Model file for the job. Use its own axes, mm. Coordinates: 2 decimals unless noted, no trailing zeros. Write each loop counter-clockwise with the first axis right and the second up, starting at its lowest first coordinate (ties: lowest second). Pieces come first, ordered by that corner, then holes.
Q1. Drill centre lines: probe 1 along Y at (x, z) = (4, -2.5); probe 2 along Z at (x, y) = (1.1, 160); probe 3 along Z at (x, y) = (3.9, 202.5). Where is each one in solid material? Low to high.
Q2. Pull direction Z, two halves, no side cores. Call faces 1 (the flat face through (2.5, 101, -75)), 2 (the flat face through (3, 104, -80)), 3 (the flat face through (0, 104, -39)): released by +Z, released by -Z, zero draft, split by the parting line, or undercut.
Q3. Band-saw the part on A-A, the plane y = 84. Write the cut outline in (x, z).
Autodesk Inventor part; units mm, degrees
ref_plane "YZ Plane" through (0, 0, 0) normal (1, 0, 0) x (0, 1, 0)
ref_plane "XZ Plane" through (0, 0, 0) normal (0, 1, 0) x (-1, 0, 0)
ref_plane "XY Plane" through (0, 0, 0) normal (0, 0, 1) x (1, 0, 0)
sketch "Sketch1" plane through (0, 0, 0) normal (1, 0, 0) x (0, 1, 0)
  line L0 (0, 0) -> (205, 0)
  line L1 (205, 0) -> (205, -70)
  line L2 (205, -70) -> (0, -70)
  line L3 (0, -70) -> (0, 0)
  circle A0 centre (40, -2.5) radius 1
  circle A1 centre (80, -2.5) radius 1
  circle A2 centre (120, -2.5) radius 1
  circle A3 centre (160, -2.5) radius 1
  line L4 (0, 0) -> (0, 5)
  circle A4 centre (202.5, -2.5) radius 1.1944
  line L5 (0, -35) -> (205, -35) construction
  point P0 (40, -67.5)
  point P1 (80, -67.5)
  point P2 (120, -67.5)
  point P3 (160, -67.5)
  point P4 (202.5, -67.5)
  dimension "d0" = 205
  dimension "d1" = 70
  dimension "d2" = 2
  dimension "d3" = 2
  dimension "d4" = 2
  dimension "d5" = 2
  dimension "d7" = 40
  dimension "d8" = 40
  dimension "d9" = 40
  dimension "d10" = 2.5
  dimension "d11" = 40
  dimension "d12" = 2.5
extrude "Extrusion1" add sketch "Sketch1" along normal blind 5 contours L0 L1 L2 L3 | A0 | A1 | A2 | A3 | A4
hole "Hole1" at (0, 202.5, -67.5) at (0, 160, -67.5) at (0, 120, -67.5) at (0, 80, -67.5) at (0, 40, -67.5) at (0, 40, -2.5) at (0, 80, -2.5) at (0, 120, -2.5) at (0, 160, -2.5) at (0, 202.5, -2.5) direction (1, 0, 0) diameter 3.242 depth 11.8
sketch "Sketch2" plane through (0, 0, -70) normal (0, 0, -1) x (-1, 0, 0)
  line L0 (0, 205) -> (0, 0)
  line L1 (-5, 205) -> (0, 205)
  line L2 (0, 205) -> (0, 0)
  line L3 (0, 0) -> (-5, 0)
  line L4 (-5, 0) -> (-5, 205)
extrude "Extrusion2" add sketch "Sketch2" along normal blind 10
sketch "Sketch3" plane through (0, 0, 0) normal (0, -1, 0) x (1, 0, 0)
  line L0 (5, 0) -> (5, -80)
  line L1 (5, -80) -> (5, -70)
  line L2 (5, -77) -> (2.5, -77)
  line L3 (2.5, -77) -> (2.5, -73)
  line L4 (2.5, -73) -> (5, -73)
  line L5 (5, -80) -> (0, -80)
  point P0 (0, 0)
  dimension "d24" = 10
  dimension "d25" = 2.5
  dimension "d26" = 4
  dimension "d27" = 3
extrude "Extrusion3" cut sketch "Sketch3" against normal up to surface (205 mm away)
properties part number "SidePanel"
Answer sheet:
1. probe 1: y = 0 to 38.38, 41.62 to 78.38, 81.62 to 118.38, 121.62 to 158.38, 161.62 to 200.88, 204.12 to 205
1. probe 2: z = -80 to -69.12, -65.88 to -4.12, -0.88 to 0
1. probe 3: z = -80 to -77, -73 to -69.12, -65.88 to -4.12, -0.88 to 0
2. face 1: undercut
2. face 2: released by -Z
2. face 3: zero draft
3. outline: (0, -80) - (5, -80) - (5, -77) - (2.5, -77) - (2.5, -73) - (5, -73) - (5, 0) - (0, 0) - close
